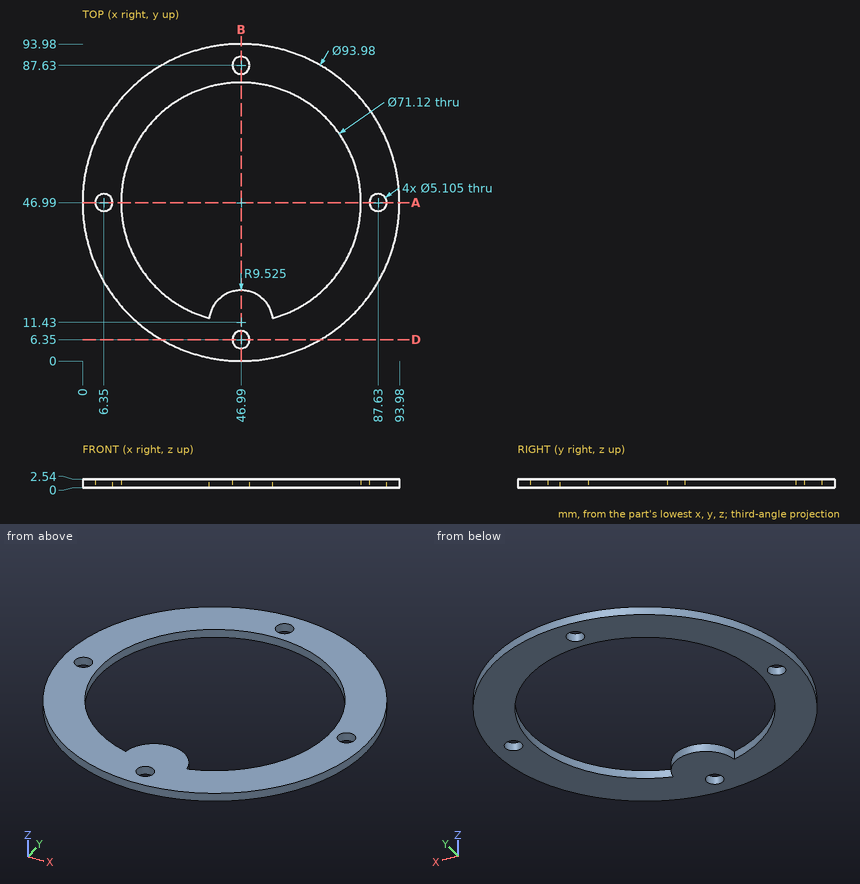
Could you check a few things on this drawing? It's one solid part, dimensions in mm from its lowest x, y, z. Give positions to 0.01 mm unless a question says otherwise; leave off trailing zeros. Write each loop counter-clockwise with the first axis right and the second up, starting at its lowest first coordinate (ties: lowest second). Pieces come first, ordered by that corner, then holes. Notation, with made-up numbers: (-31, -3.75) -> (0, -3.75) arc R22 cw to (0, 18.25) -> close; hole circle Ø1 at (-15, -7). An arc over 180 degrees is marked (long way). Answer as CSV lines item,"result". Start each with the question number.
(1) Please list where these lines run through material, in increasing order: line 1 (X direction, y = 71.5, z = 2.25) (1 decimal); line 2 (Y direction, x = 87.63, z = 1.2) (1 decimal); line 3 (Y direction, x = 21, z = 1.7).
(2) If we section it at D-D, the plane y = 6.35: Write out the boundary of the cut face in (x, z), and give its area (3 significant figures).
(3) If we section it at B-B, the plane x = 46.99: Give the number of separate pieces and of enclosed holes in the cut face.
(4) If we section it at A-A, the plane y = 46.99: Write out the boundary of the cut face in (x, z).
(5) I'm going to push flat-ended pins straight in: pin 1 Ø4 at (x, y) = (46.99, 6.35) entering from -Z; pin 2 Ø1.5 at (x, z) = (76.5, 2) entering from +Y; pin 3 Ø1 at (y, z) = (29, 2) entering from +X. Where does each tip first touch, or does it pass through?
Answer list:
1,line 1,"6.9 to 21.2, 72.8 to 87.1"
1,line 2,"23.4 to 44.4, 49.5 to 70.6"
1,line 3,"7.84 to 22.72, 71.26 to 86.14"
2,outline,"(23.4, 0) -> (44.44, 0) -> (44.44, 2.54) -> (23.4, 2.54) -> close; (49.54, 0) -> (70.58, 0) -> (70.58, 2.54) -> (49.54, 2.54) -> close"
2,area,"107 mm^2"
3,separate pieces,"4"
3,enclosed holes,"0"
4,outline,"(0, 0) -> (3.8, 0) -> (3.8, 2.54) -> (0, 2.54) -> close; (8.9, 0) -> (11.43, 0) -> (11.43, 2.54) -> (8.9, 2.54) -> close; (82.55, 0) -> (85.08, 0) -> (85.08, 2.54) -> (82.55, 2.54) -> close; (90.18, 0) -> (93.98, 0) -> (93.98, 2.54) -> (90.18, 2.54) -> close"
5,pin 1,"through"
5,pin 2,"y = 84.15"
5,pin 3,"x = 90.6"
